from build123d import *

# Parameters (mm, degrees)
SKETCH1_R               = 22
BOSS_EXTRUDE1_DEPTH     = 10
CUT_EXTRUDE1_DEPTH      = 3.2
CUT_EXTRUDE2_DEPTH      = 32.847134879
CUT_EXTRUDE2_DEPTH_BACK = 6
SKETCH3_W               = 30
SKETCH3_H               = 31
CUT_EXTRUDE3_DEPTH      = 6
CUT_EXTRUDE3_DEPTH_BACK = 50.064141692
FILLET1_R               = 3
FILLET2_R               = 1.5
FILLET3_R               = 5
CUT_EXTRUDE4_DEPTH      = 32.847135017
CUT_EXTRUDE4_DEPTH_BACK = 4
CUT_EXTRUDE6_DEPTH      = 2.3
SKETCH10_R              = 21
CUT_EXTRUDE5_DEPTH      = 1.5


with BuildPart() as part:
    # Sketch1 → Boss-Extrude1 (new body)
    with BuildSketch(Plane(origin=(0, 0, 0), x_dir=(1, 0, 0), z_dir=(0, 1, 0))):
        with Locations(Location((0, 0, 0), (0, 0, 270))):
            Circle(SKETCH1_R)
    extrude(amount=BOSS_EXTRUDE1_DEPTH)

    # Sketch2 → Cut-Extrude1 (cut)
    with BuildSketch(Plane(origin=(0, 10, 0), x_dir=(1, 0, 0), z_dir=(0, 1, 0))):
        with BuildLine():
            Line((4, 19.595917942), (3.8, 18.616122045))
            ThreePointArc((3.8, 18.616122045), (0, -19), (-3.8, 18.616122045))
            Line((-3.8, 18.616122045), (-4, 19.595917942))
            ThreePointArc((-4, 19.595917942), (0, 20), (4, 19.595917942))
        make_face()
        with BuildLine():
            ThreePointArc((12.899684367, -13.949843843), (0, -19), (-12.899684367, -13.949843843))
            Line((-12.899684367, -13.949843843), (-5.6, -20.7))
            Line((-5.6, -20.7), (5.6, -20.7))
            Line((5.6, -20.7), (12.899684367, -13.949843843))
        make_face()
    extrude(amount=-CUT_EXTRUDE1_DEPTH, mode=Mode.SUBTRACT)

    # Sketch3 → Cut-Extrude2 (cut, two sides: drawn at the far end of the back side and taken through both)
    with BuildSketch(Plane(origin=(0, 6.8, 0), x_dir=(1, 0, 0), z_dir=(0, 1, 0)).offset(-CUT_EXTRUDE2_DEPTH_BACK)):
        Rectangle(SKETCH3_W, SKETCH3_H)
    extrude(amount=CUT_EXTRUDE2_DEPTH + CUT_EXTRUDE2_DEPTH_BACK, mode=Mode.SUBTRACT)

    # Sketch5 → Cut-Extrude3 (cut, two sides: drawn at the far end of the back side and taken through both)
    with BuildSketch(Plane(origin=(0, 0, 20.7), x_dir=(-1, 0, 0), z_dir=(0, 0, -1)).offset(-CUT_EXTRUDE3_DEPTH_BACK)):
        with BuildLine():
            Line((-2.75, 9.2), (2.75, 9.2))
            ThreePointArc((2.75, 9.2), (4.65, 7.3), (2.75, 5.4))
            Line((2.75, 5.4), (-2.75, 5.4))
            ThreePointArc((-2.75, 5.4), (-4.65, 7.3), (-2.75, 9.2))
        make_face()
    extrude(amount=CUT_EXTRUDE3_DEPTH + CUT_EXTRUDE3_DEPTH_BACK, mode=Mode.SUBTRACT)

    # Fillet1
    fillet1_edges = [part.edges().sort_by_distance(p)[0] for p in [
        (-15, 0.8, 0),
        (15, 0.8, 0),
    ]]
    fillet(fillet1_edges, radius=FILLET1_R)

    # Fillet2
    fillet2_edges = [part.edges().sort_by_distance(p)[0] for p in [
        (0, 0.8, 15.5),
        (0, 0.8, -15.5),
        (14.121320344, 1.678679656, 15.5),
        (-14.121320344, 1.678679656, 15.5),
        (14.121320344, 1.678679656, -15.5),
        (-14.121320344, 1.678679656, -15.5),
        (-15, 6.9, -15.5),
        (-15, 6.9, 15.5),
        (15, 6.9, 15.5),
        (15, 6.9, -15.5),
    ]]
    fillet(fillet2_edges, radius=FILLET2_R)

    # Fillet3
    fillet3_edges = [part.edges().sort_by_distance(p)[0] for p in [
        (0, 0, -22),
    ]]
    fillet(fillet3_edges, radius=FILLET3_R)

    # Sketch6 → Cut-Extrude4 (cut, two sides: drawn at the far end of the back side and taken through both)
    with BuildSketch(Plane(origin=(0, 6.8, 0), x_dir=(1, 0, 0), z_dir=(0, 1, 0)).offset(-CUT_EXTRUDE4_DEPTH_BACK)):
        Polygon((16.5, -3.3), (16.5, -4.3), (19.5, -4.3), (19.5, -3.3), (20.5, -3.3), (20.5, 4.7), (19.9, 4.7), (16.1, 4.7), (15.5, 4.7), (15.5, -3.3), align=None)
        with BuildLine():
            ThreePointArc((15, 5.8), (15.777817459, 5.477817459), (16.1, 4.7))
            Line((16.1, 4.7), (19.9, 4.7))
            ThreePointArc((19.9, 4.7), (18.464823228, 8.164823228), (15, 9.6))
            Line((15, 9.6), (15, 5.8))
        make_face()
    extrude(amount=CUT_EXTRUDE4_DEPTH + CUT_EXTRUDE4_DEPTH_BACK, mode=Mode.SUBTRACT)

    # Sketch11 → Cut-Extrude6 (cut)
    with BuildSketch(Plane.XY.offset(4.3)):
        with BuildLine():
            Line((15.7, 5.1), (15.7, 10))
            Line((15.7, 10), (20.3, 10))
            Line((20.3, 10), (20.3, 5.1))
            ThreePointArc((20.3, 5.1), (18, 2.8), (15.7, 5.1))
        make_face()
    extrude(amount=CUT_EXTRUDE6_DEPTH, mode=Mode.SUBTRACT)

    # Sketch10 → Cut-Extrude5 (cut)
    with BuildSketch(Plane(origin=(0, 10, 0), x_dir=(1, 0, 0), z_dir=(0, 1, 0))):
        Circle(SKETCH10_R)
        with BuildLine():
            Line((19.5, -4.3), (19.532280973, -4.3))
            ThreePointArc((19.532280973, -4.3), (-19.635443226, 3.801232604), (19.725871337, -3.3))
            Line((19.725871337, -3.3), (19.5, -3.3))
            Line((19.5, -3.3), (19.5, -4.3))
        make_face(mode=Mode.SUBTRACT)
    extrude(amount=-CUT_EXTRUDE5_DEPTH, mode=Mode.SUBTRACT)


solid = part.part
Geometry: final body of the model. Coordinates: model frame, mm. A direction names the side the tool comes from. Give positions to 0.01 mm unless a question says otherwise; leave off trailing zeros. Loops run counter-clockwise (first coordinate to the right, second up) from the corner with the lowest first, then second, coordinate; pieces in that order, holes last. Notation, with made-up numbers: M 6.5,-4.5 L 65.5,-4.5 A8 cw 65.5,10.5 Z; hole C 64.25,32 d2. An arc over 180 degrees is marked long. Put each result on its own line as item: value. Start each with the question number.
1) Ray query, line 1 along X through (y, z) = (9, 0.5); line 2 along Z through (x, y) = (-11, 9); line 3 along X through (y, z) = (5, -2). Return the intervals inside material, ascending.
2) Cut plane B-B (y = 6.25). Output: boundary loops of the cut face in (x, z), then the cut area to 3 significant figures.
3) Access query for faces 4 (the cylindrical face through (-21.477, 7.465, -4.769)), 5 (the flat face through (0, 5, 15.5)). Directions: +Z, -Z, +X, -X, +Y, -Y. A direction counts if a zero-diameter tool reaches every point of the face in a straight line with its end or side. Return the directions, or none.
4) Contact query for flat-ended pins moving along their axis: pin 1 (2 mm diameter, centred on y = 7.5, z = 6, fed in from -X); pin 2 (6 mm diameter, centred on x = 6, y = 8, fed in from -Z); pin 3 (1.6 mm diameter, centred on x = -8, z = 19, fed in from +Y); pin 4 (5 mm diameter, centred on x = -11.5, y = 2, fed in from -Z). Output: stop coordinate, or through.
5) Cut plane A-A (x = 0). Output: boundary loops of the cut face in (y, z), then the cut area to 3 significant figures.
6) Pull-direction query (Y, two-part tool) for faces 1 (the cylindrical face through (4.18, 6.05, 19.41)), 2 (the cylindrical face through (16.622, 8.422, 9.203)), 3 (the flat face through (15.6, 8.5, 13.8)); classes: pulls with the +Y half, pulls with the -Y half, needs draft (parallel to the pull), parting line crosses it, or undercut.
Verdict:
1. line 1: -21.99 to -20.99, -19.99 to -18.99, 20.99 to 21.99
1. line 2: -19.05 to -17.89, -16.7 to -15.5, 15.71 to 16.7, 17.89 to 19.05
1. line 3: -21.91 to -15, 15 to 15.5, 20.5 to 21.91
2. outline: M -15,-14 L -15,14 A1.5 cw -13.5,15.5 L -4.33,15.5 L -4.33,21.57 A22 ccw long 4.33,21.57 L 4.33,15.5 L 13.5,15.5 A1.5 cw 15,14 L 15,-5.8 A1.1 ccw 16.1,-4.7 L 15.5,-4.7 L 15.5,3.3 L 16.5,3.3 L 16.5,4.3 L 15.7,4.3 L 15.7,6.6 L 20.3,6.6 L 20.3,4.3 L 19.5,4.3 L 19.5,3.3 L 20.5,3.3 L 20.5,-4.7 L 19.9,-4.7 A4.9 cw 15,-9.6 L 15,-14 A1.5 cw 13.5,-15.5 L -13.5,-15.5 A1.5 cw Z
2. area: 466 mm2
3. face 4: +Y, -Y
3. face 5: +Y
4. pin 1: x = -21.42
4. pin 2: z = -21.79
4. pin 3: y = 10
4. pin 4: z = -19.59
5. outline: M 0,-17 A5 ccw 5,-22 L 10,-22 L 10,-21 L 8.5,-21 L 8.5,-20 L 6.8,-20 L 6.8,-15.5 L 2.3,-15.5 A1.5 cw 0.8,-14 L 0.8,14 A1.5 cw 2.3,15.5 L 5.4,15.5 L 5.4,22 L 5,22 A5 ccw 0,17 Z; M 9.2,21 L 10,21 L 10,22 L 9.2,22 Z
5. area: 100 mm2
6. face 1: undercut
6. face 2: needs draft
6. face 3: pulls with the +Y half
